Here's how the part is built. I have some questions about the finished solid (model axes, mm). A direction names the side the tool comes from. Round coordinates to 2 decimals unless told otherwise and drop trailing zeros. Order: outer loops, then holes, each group sorted by start corner. A loop starts at its lowest first (then second) coordinate and runs counter-clockwise, first axis right, second up. Notation, with made-up numbers: (79, 36) - (117, 36) arc R21 cw to (117, 73) - close; hole circle Ø1 at (39, 69). An arc over 180 degrees is marked (long way). Answer as a JSON object with one key per item and string values.
```python
from build123d import *

# Parameters (mm, degrees)
ESBO_O1_W                = 130
ESBO_O1_H                = 130
RESSALTO_EXTRUS_O1_DEPTH = 15
ESBO_O2_R                = 4.2
CORTE_EXTRUS_O1_DEPTH    = 12
ESBO_O3_R                = 12.5
CORTE_EXTRUS_O2_DEPTH    = 16
ESBO_O4_R                = 11.15
CORTE_EXTRUS_O3_DEPTH    = 7
ESBO_O5_W                = 25
ESBO_O5_H                = 50
CORTE_EXTRUS_O4_DEPTH    = 16
FILETE1_R                = 5
ESBO_O6_R                = 5
CORTE_EXTRUS_O5_DEPTH    = 6.5
ESBO_O7_R                = 3
CORTE_EXTRUS_O6_DEPTH    = 9.5
ESBO_O8_W                = 15
ESBO_O8_H                = 15
CORTE_EXTRUS_O7_DEPTH    = 16
ESBO_O9_R                = 2
CORTE_EXTRUS_O8_DEPTH    = 10
ESBO_O10_R               = 2
CORTE_EXTRUS_O9_DEPTH    = 10
ESBO_O11_R               = 2
CORTE_EXTRUS_O10_DEPTH   = 10
ESBO_O12_R               = 2
CORTE_EXTRUS_O11_DEPTH   = 10
FILETE2_R                = 5
CORTE_EXTRUS_O12_DEPTH   = 16
ESBO_O14_R               = 2
CORTE_EXTRUS_O13_DEPTH   = 10
FILETE4_R                = 5
FILETE5_R                = 2.5


with BuildPart() as part:
    # Esboço1 → Ressalto-extrusão1 (new body)
    with BuildSketch(Plane(origin=(0, 0, 0), x_dir=(1, 0, 0), z_dir=(0, 1, 0))):
        Rectangle(ESBO_O1_W, ESBO_O1_H)
    extrude(amount=RESSALTO_EXTRUS_O1_DEPTH)

    # Esboço2 → Corte-extrusão1 (cut)
    with BuildSketch(Plane(origin=(0, 15, 0), x_dir=(1, 0, 0), z_dir=(0, 1, 0))):
        with Locations((-30, 5)):
            Circle(ESBO_O2_R)
        with Locations((30, 5)):
            Circle(ESBO_O2_R)
        with Locations((30, -55)):
            Circle(ESBO_O2_R)
        with Locations((-30, -55)):
            Circle(ESBO_O2_R)
        with Locations((-30, 40)):
            Circle(ESBO_O2_R)
        with Locations((30, 40)):
            Circle(ESBO_O2_R)
    extrude(amount=-CORTE_EXTRUS_O1_DEPTH, mode=Mode.SUBTRACT)

    # Esboço3 → Corte-extrusão2 (cut, through all)
    with BuildSketch(Plane(origin=(0, 15, 0), x_dir=(1, 0, 0), z_dir=(0, 1, 0))):
        with Locations((0, -25)):
            Circle(ESBO_O3_R)
    extrude(amount=-CORTE_EXTRUS_O2_DEPTH, mode=Mode.SUBTRACT)

    # Esboço4 → Corte-extrusão3 (cut)
    with BuildSketch(Plane(origin=(0, 15, 0), x_dir=(1, 0, 0), z_dir=(0, 1, 0))):
        with Locations((0, 40)):
            Circle(ESBO_O4_R)
    extrude(amount=-CORTE_EXTRUS_O3_DEPTH, mode=Mode.SUBTRACT)

    # Esboço5 → Corte-extrusão4 (cut, through all)
    with BuildSketch(Plane(origin=(0, 15, 0), x_dir=(1, 0, 0), z_dir=(0, 1, 0))):
        with Locations((-52.5, 40)):
            Rectangle(ESBO_O5_W, ESBO_O5_H)
        with Locations((52.5, 40)):
            Rectangle(ESBO_O5_W, ESBO_O5_H)
    extrude(amount=-CORTE_EXTRUS_O4_DEPTH, mode=Mode.SUBTRACT)

    # Filete1
    filete1_edges = [part.edges().sort_by_distance(p)[0] for p in [
        (-40, 7.5, -65),
        (40, 7.5, -65),
    ]]
    fillet(filete1_edges, radius=FILETE1_R)

    # Esboço6 → Corte-extrusão5 (cut)
    with BuildSketch(Plane(origin=(0, 15, 0), x_dir=(1, 0, 0), z_dir=(0, 1, 0))):
        with Locations((-55, 5)):
            Circle(ESBO_O6_R)
        with Locations((55, 5)):
            Circle(ESBO_O6_R)
        with Locations((55, -55)):
            Circle(ESBO_O6_R)
        with Locations((-55, -55)):
            Circle(ESBO_O6_R)
    extrude(amount=-CORTE_EXTRUS_O5_DEPTH, mode=Mode.SUBTRACT)

    # Esboço7 → Corte-extrusão6 (cut, through all)
    with BuildSketch(Plane(origin=(0, 8.5, 0), x_dir=(1, 0, 0), z_dir=(0, 1, 0))):
        with Locations((-55, 5)):
            Circle(ESBO_O7_R)
        with Locations((55, 5)):
            Circle(ESBO_O7_R)
        with Locations((55, -55)):
            Circle(ESBO_O7_R)
        with Locations((-55, -55)):
            Circle(ESBO_O7_R)
    extrude(amount=-CORTE_EXTRUS_O6_DEPTH, mode=Mode.SUBTRACT)

    # Esboço8 → Corte-extrusão7 (cut, through all)
    with BuildSketch(Plane(origin=(0, 15, 0), x_dir=(1, 0, 0), z_dir=(0, 1, 0))):
        with Locations((0, 65)):
            Rectangle(ESBO_O8_W, ESBO_O8_H)
    extrude(amount=-CORTE_EXTRUS_O7_DEPTH, mode=Mode.SUBTRACT)

    # Esboço9 → Corte-extrusão8 (cut)
    with BuildSketch(Plane(origin=(0, 0, -57.5), x_dir=(-1, 0, 0), z_dir=(0, 0, -1))):
        with Locations((0, 11.5)):
            Circle(ESBO_O9_R)
    extrude(amount=-CORTE_EXTRUS_O8_DEPTH, mode=Mode.SUBTRACT)

    # Esboço10 → Corte-extrusão9 (cut)
    with BuildSketch(Plane.ZY.offset(40)):
        with Locations((-40, 9)):
            Circle(ESBO_O10_R)
    extrude(amount=-CORTE_EXTRUS_O9_DEPTH, mode=Mode.SUBTRACT)

    # Esboço11 → Corte-extrusão10 (cut)
    with BuildSketch(Plane(origin=(40, 0, 0), x_dir=(0, 0, -1), z_dir=(1, 0, 0))):
        with Locations((40, 9)):
            Circle(ESBO_O11_R)
    extrude(amount=-CORTE_EXTRUS_O10_DEPTH, mode=Mode.SUBTRACT)

    # Esboço12 → Corte-extrusão11 (cut)
    with BuildSketch(Plane.XY.offset(65)):
        with Locations((-30, 9)):
            Circle(ESBO_O12_R)
        with Locations((30, 9)):
            Circle(ESBO_O12_R)
    extrude(amount=-CORTE_EXTRUS_O11_DEPTH, mode=Mode.SUBTRACT)

    # Filete2
    filete2_edges = [part.edges().sort_by_distance(p)[0] for p in [
        (-40, 7.5, -15),
        (40, 7.5, -15),
    ]]
    fillet(filete2_edges, radius=FILETE2_R)

    # Esboço13 → Corte-extrusão12 (cut, through all)
    with BuildSketch(Plane(origin=(0, 15, 0), x_dir=(1, 0, 0), z_dir=(0, 1, 0))):
        Polygon((-7.5, 57.5), (-20, 57.5), (-20, 50), (-40, 50), (-40, 57.5), (-40, 65), (-7.5, 65), align=None)
        Polygon((7.5, 57.5), (7.5, 65), (40, 65), (40, 57.5), (40, 50), (20, 50), (20, 57.5), align=None)
    extrude(amount=-CORTE_EXTRUS_O12_DEPTH, mode=Mode.SUBTRACT)

    # Esboço14 → Corte-extrusão13 (cut)
    with BuildSketch(Plane(origin=(0, 0, -50), x_dir=(-1, 0, 0), z_dir=(0, 0, -1))):
        with Locations((-30, 9)):
            Circle(ESBO_O14_R)
        with Locations((30, 9)):
            Circle(ESBO_O14_R)
    extrude(amount=-CORTE_EXTRUS_O13_DEPTH, mode=Mode.SUBTRACT)

    # Filete4
    filete4_edges = [part.edges().sort_by_distance(p)[0] for p in [
        (-40, 7.5, -50),
        (40, 7.5, -50),
    ]]
    fillet(filete4_edges, radius=FILETE4_R)

    # Filete5
    filete5_edges = [part.edges().sort_by_distance(p)[0] for p in [
        (-20, 7.5, -57.5),
        (-20, 7.5, -50),
        (20, 7.5, -57.5),
        (20, 7.5, -50),
    ]]
    fillet(filete5_edges, radius=FILETE5_R)


solid = part.part
```
1. If I drill on L1, parallel to Z at x = -55, y = 13.5; L2, parallel to X at y = 9, z = 63; L3, parallel to X at y = 6, z = -40, over which ranges is the centre line in solid material (lowest first)? Write a range as [from, to].
Responses:
{"L1": "[-15, -10], [0, 50], [60, 65]", "L2": "[-65, -32], [-28, 28], [32, 65]", "L3": "[-40, -34.2], [-25.8, 25.8], [34.2, 40]"}
2. Imagine slicing it at B-B (x = 0). List the corners of the cut face in (y, z) for me, plus the area to 3 significant figures.
Responses:
{"outline": "(0, -57.5) - (9.5, -57.5) - (9.5, -51.15) - (8, -51.15) - (8, -28.85) - (15, -28.85) - (15, 12.5) - (0, 12.5) - close; (0, 37.5) - (15, 37.5) - (15, 65) - (0, 65) - close; (13.5, -57.5) - (15, -57.5) - (15, -51.15) - (13.5, -51.15) - close", "area": "1,280 mm2"}
3. For P1, Ø1.5, axis at y = 8.5, z = -19, coming from the -X side; P2, Ø4, axis at x = -27.5, y = 7, coming from the -Z side; P3, Ø6, axis at x = 27.5, z = -15, coming from the -Y side; P4, Ø9.5, axis at x = -55, z = -5, coming from the +Y side, each with a flat end and sliding along its axis, tell me the tip position at first contact or that it passes through.
Responses:
{"P1": "x = -40.32", "P2": "z = -50", "P3": "y = 0", "P4": "y = 8.5"}
4. Imagine slicing it at D-D (y = 5). Give the number of separate pieces and of enclosed holes in the cut face, plus the area to 3 significant figures.
Responses:
{"separate pieces": "1", "enclosed holes": "11", "area": "12,600 mm2"}
5. Imagine slicing it at A-A (z = 21.5). List the corners of the cut face in (x, y) for me.
Responses:
{"outline": "(-65, 0) - (-12, 0) - (-12, 15) - (-65, 15) - close; (12, 0) - (65, 0) - (65, 15) - (12, 15) - close"}
6. Thinking about a two-plate mould opening in X: for faces 4 (the face through (41, 7, -17)), 5 (the face through (-51.7, 8.5, 54.9)), 6 (the face through (-1, 7, 65)), 7 (the face through (-42, 7, -16)), which applies, pulls with the +X half, pulls with the -X half, needs draft (parallel to the pull), parting line crosses it, or undercut?
Responses:
{"face 4": "pulls with the +X half", "face 5": "undercut", "face 6": "needs draft", "face 7": "pulls with the -X half"}
7. Imagine slicing it at C-C (z = -40). List the corners of the cut face in (x, y) for me, plus the area to 3 significant figures.
Responses:
{"outline": "(-40, 0) - (40, 0) - (40, 7) - (34.2, 7) - (34.2, 3) - (25.8, 3) - (25.8, 15) - (11.15, 15) - (11.15, 8) - (-11.15, 8) - (-11.15, 15) - (-25.8, 15) - (-25.8, 3) - (-34.2, 3) - (-34.2, 7) - (-40, 7) - close; (-40, 11) - (-34.2, 11) - (-34.2, 15) - (-40, 15) - close; (34.2, 11) - (40, 11) - (40, 15) - (34.2, 15) - close", "area": "796 mm2"}
8. For faces 1 (the face through (-51.7, 8.5, -5.1)), 2 (the face through (0.26, 13.483, -54.278)), 3 (the face through (-40, 8, -32)), which set-ups out of +Z, -Z, +X, -X, +Y, -Y let a thin tool reach every point of the face, with its end or its side?
Responses:
{"face 1": "+Y", "face 2": "-Z", "face 3": "-Z, -X, +Y, -Y"}
